Check sheet for the drawn part. Datum: minimum x, y, z corner. Units: mm. Give positions to 0.01 mm unless a question says otherwise; leave off trailing zeros. Order: outer loops, then holes, each group sorted by start corner. A loop starts at its lowest first (then second) coordinate and runs counter-clockwise, first axis right, second up. Notation, with made-up numbers: (30, -10.5) - (60, -10.5) arc R30 cw to (60, 12.5) - close; hole circle Ø8 at (-12.5, -9.5). An arc over 180 degrees is marked (long way). Answer as a JSON object with one key per item and string values. Group by question number.
(1) Section check B-B (x = 10). Record the boundary of the cut face in (y, z), then the cut area to 4 significant figures.
(2) Section check C-C (y = 4.35). Record the boundary of the cut face in (x, z).
(3) Mould release check, pull along Z, two halves, no side actions. Record for the marked faces 1, 2 and 3: +Z half, -Z half, draft (parallel to the pull), parting line (faces both ways), or undercut.
(4) Section check D-D (z = 8). Record the boundary of the cut face in (x, y).
(5) Thickness scan on line 1 (X direction, y = 4.15, z = 10); line 2 (X direction, y = 1.45, z = 10). Record the ranges inside material, lowest first.
(6) Depth check by flat-ended pin: pin 1 Ø6.5 at (x, z) = (9, 9.5) entering from +Y; pin 2 Ø1 at (y, z) = (0.5, 4.5) entering from -X. Enter the tip coordinate at first touch or a pass-through.
(7) Section check A-A (z = 10). Record the boundary of the cut face in (x, y).
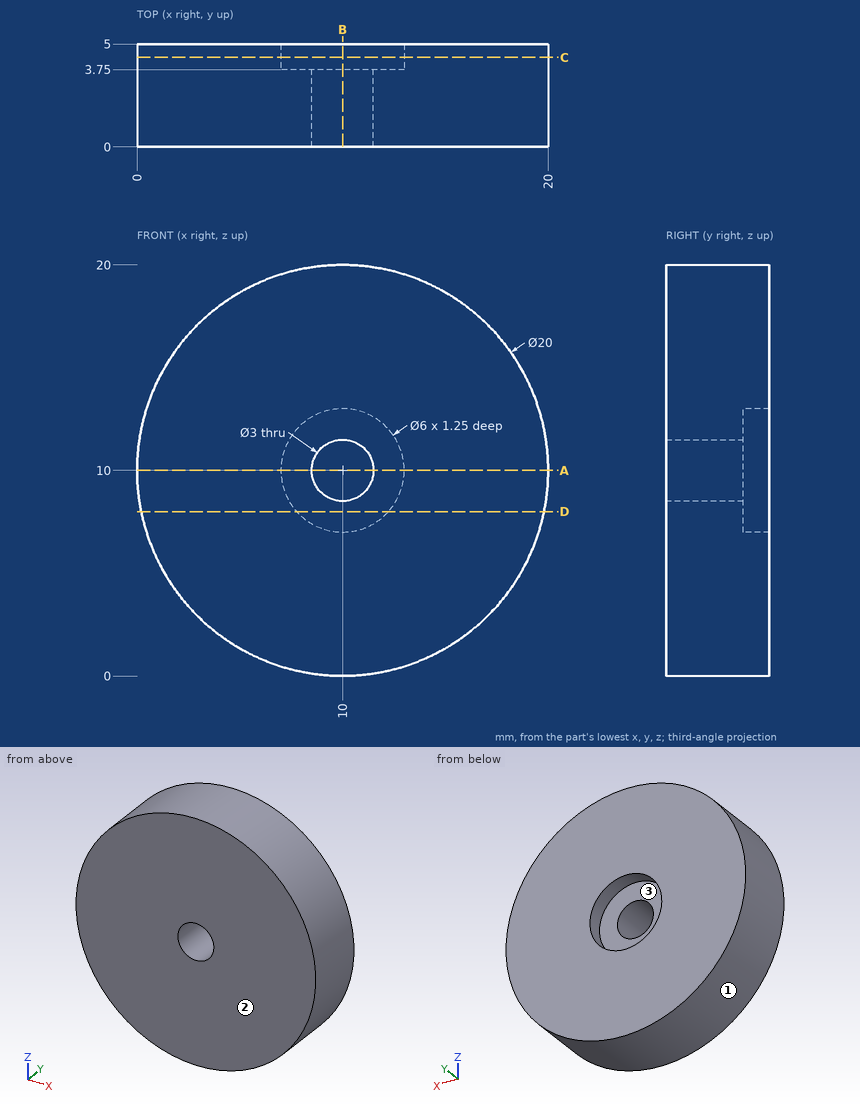
Solutions:
{
 "1": {"outline": "(0, 0) - (5, 0) - (5, 7) - (3.75, 7) - (3.75, 8.5) - (0, 8.5) - close; (0, 11.5) - (3.75, 11.5) - (3.75, 13) - (5, 13) - (5, 20) - (0, 20) - close", "area": "81.25 mm2"},
 "2": {"outline": "circle Ø20 at (10, 10); hole circle Ø6 at (10, 10)"},
 "3": {"face 1": "parting line", "face 2": "draft", "face 3": "undercut"},
 "4": {"outline": "(0.2, 0) - (19.8, 0) - (19.8, 5) - (12.24, 5) - (12.24, 3.75) - (7.76, 3.75) - (7.76, 5) - (0.2, 5) - close"},
 "5": {"line 1": "x = 0 to 7, 13 to 20", "line 2": "x = 0 to 8.5, 11.5 to 20"},
 "6": {"pin 1": "stops at y = 5", "pin 2": "stops at x = 1.34"},
 "7": {"outline": "(0, 0) - (8.5, 0) - (8.5, 3.75) - (7, 3.75) - (7, 5) - (0, 5) - close; (11.5, 0) - (20, 0) - (20, 5) - (13, 5) - (13, 3.75) - (11.5, 3.75) - close"}
}
